Geometry check sheet. Reference: the model listing, model coordinates, mm. Face numbers are marked on the shaded views. Coordinates: 2 decimals unless noted, no trailing zeros. Write each loop counter-clockwise with the first axis right and the second up, starting at its lowest first coordinate (ties: lowest second). Pieces come first, ordered by that corner, then holes. Notation, with made-up numbers: (-7, -20) -> (18, -20) arc R15 cw to (18, -4) -> close; hole circle Ø2 at (40, -35.75). An arc over 180 degrees is marked (long way). Answer in a Markdown table with one row per item. Add a question column.
Q1. Section check D-D, the plane y = 1.55. Record the boundary of the cut face in (x, z), and give its area (3 significant figures).
Q2. Release check for a two-part mould opening along Y. For the marked faces 1, 2 and 3 record: pulls with the +Y half, pulls with the -Y half, needs draft (parallel to the pull), parting line crosses it, or undercut.
Q3. Section check C-C, the plane z = 1.5. Record the boundary of the cut face in (x, y), and give its area (3 significant figures).
Q4. Section check A-A, the plane z = -7. Record the boundary of the cut face in (x, y), and give its area (3 significant figures).
Q5. Section check B-B, the plane x = -5. Record the boundary of the cut face in (y, z).
Q6. Thickness scan on line 1 (Z direction, x = -5, y = 0.9); line 2 (Z direction, x = -5, y = -1.9); line 3 (X direction, y = 1.7, z = -7). Record the ranges inside material, lowest first.
```python
from build123d import *

# Parameters (mm, degrees)
BOSS_EXTRUDE1_DEPTH                                 = 11
FILLET1_R                                           = 1
CHAMFER1_SIZE                                       = 1
CUT_EXTRUDE1_DEPTH                                  = 25.50510151
CSK_FOR_M2_5_CROSS_RECESSED_RAISED_CTSK_D           = 2.9
CSK_FOR_M2_5_CROSS_RECESSED_RAISED_CTSK_CSINK_D     = 5.4
CSK_FOR_M2_5_CROSS_RECESSED_RAISED_CTSK_CSINK_ANGLE = 90


with BuildPart() as part:
    # Sketch1 → Boss-Extrude1 (new, symmetric)
    with BuildSketch(Plane.XY):
        Polygon((-10.5, 2.5), (-8, 0), (-10.5, -2.5), (0, -2.5), (0, 2.5), align=None)
    extrude(amount=BOSS_EXTRUDE1_DEPTH, both=True)

    # Fillet1
    fillet1_edges = [part.edges().sort_by_distance(p)[0] for p in [
        (-8, 0, 0),
    ]]
    fillet(fillet1_edges, radius=FILLET1_R)

    # Chamfer1
    chamfer1_edges = [part.edges().sort_by_distance(p)[0] for p in [
        (-10.5, -2.5, 0),
    ]]
    chamfer(chamfer1_edges, length=CHAMFER1_SIZE)

    # Sketch2 → Cut-Extrude1 (cut, through all)
    with BuildSketch(Plane.XY.offset(11)):
        Polygon((-10.5, 2.5), (-10, 2), (-10, 2.5), align=None)
    extrude(amount=-CUT_EXTRUDE1_DEPTH, mode=Mode.SUBTRACT)

    # CSK for M2.5 Cross recessed raised CTSK head wood screws1 (through all)
    with Locations(Plane(origin=(-5, -2.5, 7), x_dir=(-1, 0, 0), z_dir=(0, -1, 0))):
        with Locations((0, 0), (0, 14)):
            CounterSinkHole(CSK_FOR_M2_5_CROSS_RECESSED_RAISED_CTSK_D / 2, CSK_FOR_M2_5_CROSS_RECESSED_RAISED_CTSK_CSINK_D / 2, counter_sink_angle=CSK_FOR_M2_5_CROSS_RECESSED_RAISED_CTSK_CSINK_ANGLE)


solid = part.part
```
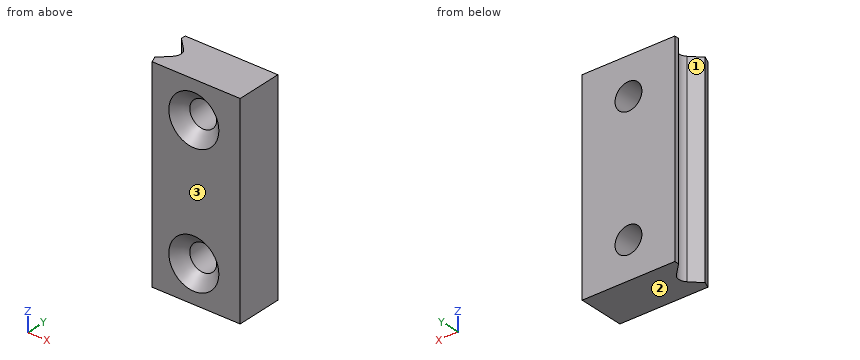
Calculated:
| question | item | result |
|---|---|---|
| 1 | outline | (-9.55, -11) -> (0, -11) -> (0, 11) -> (-9.55, 11) -> close; hole circle Ø2.9 at (-5, -7); hole circle Ø2.9 at (-5, 7) |
| 1 | area | 197 mm² |
| 2 | face 1 | undercut |
| 2 | face 2 | needs draft |
| 2 | face 3 | pulls with the -Y half |
| 3 | outline | (-10, 2) -> (-8.71, 0.71) arc R1 cw to (-8.71, -0.71) -> (-9.79, -1.79) -> (-9.5, -2.5) -> (0, -2.5) -> (0, 2.5) -> (-10, 2.5) -> close |
| 3 | area | 46.0 mm² |
| 4 | outline | (-10, 2) -> (-8.71, 0.71) arc R1 cw to (-8.71, -0.71) -> (-9.79, -1.79) -> (-9.5, -2.5) -> (-7.7, -2.5) -> (-6.45, -1.25) -> (-6.45, 2.5) -> (-10, 2.5) -> close; (-3.55, -1.25) -> (-2.3, -2.5) -> (0, -2.5) -> (0, 2.5) -> (-3.55, 2.5) -> close |
| 4 | area | 29.9 mm² |
| 5 | outline | (-2.5, -11) -> (2.5, -11) -> (2.5, -8.45) -> (-1.25, -8.45) -> (-2.5, -9.7) -> close; (-2.5, -4.3) -> (-1.25, -5.55) -> (2.5, -5.55) -> (2.5, 5.55) -> (-1.25, 5.55) -> (-2.5, 4.3) -> close; (-2.5, 9.7) -> (-1.25, 8.45) -> (2.5, 8.45) -> (2.5, 11) -> (-2.5, 11) -> close |
| 6 | line 1 | z = -11 to -8.45, -5.55 to 5.55, 8.45 to 11 |
| 6 | line 2 | z = -11 to -9.1, -4.9 to 4.9, 9.1 to 11 |
| 6 | line 3 | x = -9.7 to -6.45, -3.55 to 0 |
